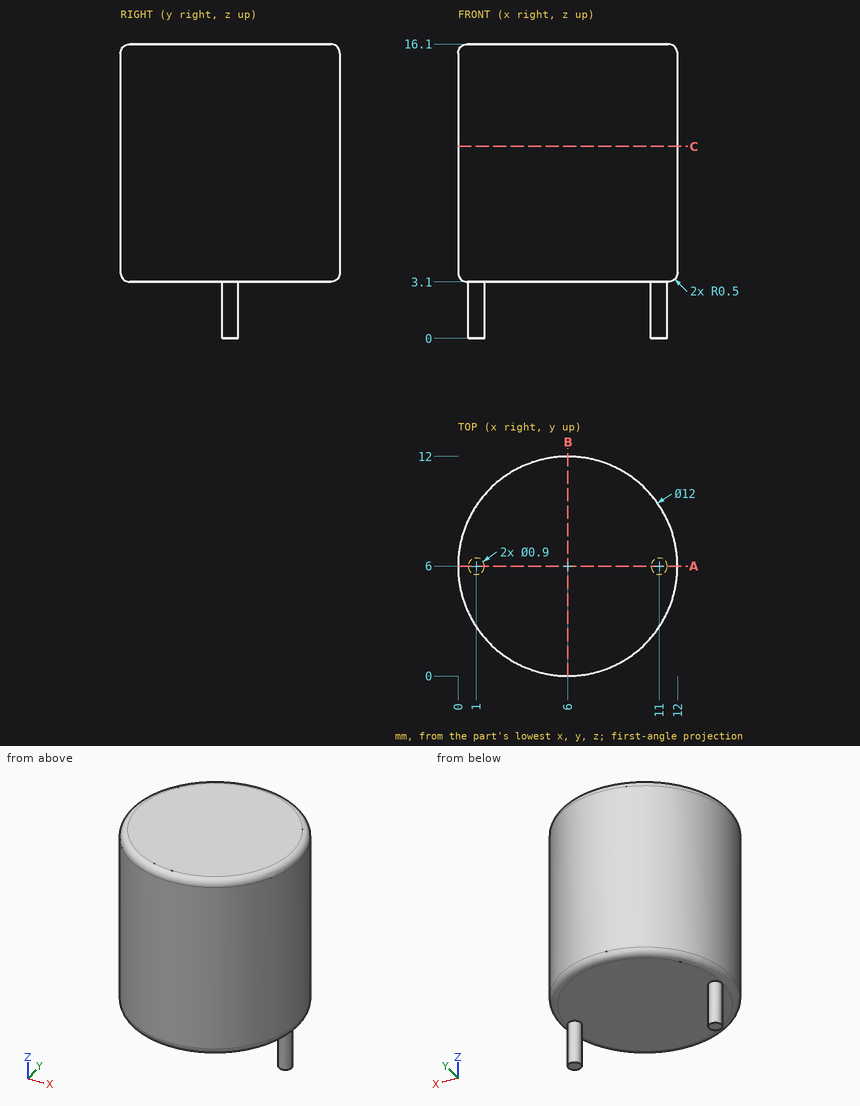
Can you work these out from the drawing? Everything is in mm from the part's minimum corner. Give positions to 0.01 mm unless a question says otherwise; leave off trailing zeros. Loops run counter-clockwise (first coordinate to the right, second up) from the corner with the lowest first, then second, coordinate; pieces in that order, holes last. Notation, with made-up numbers: (58.25, 15) - (82.25, 15) arc R23 ccw to (82.25, 40) - close; hole circle Ø3 at (-22, 54.25). An arc over 180 degrees is marked (long way). Answer as a JSON object with one key per item and string values.
Q1. Imagine slicing it at A-A on y = 6. Write out the boundary of the cut face in (x, z).
Geometry says:
{"outline": "(0, 3.6) arc R0.5 ccw to (0.5, 3.1) - (0.55, 3.1) - (0.55, 0) - (1.45, 0) - (1.45, 3.1) - (10.55, 3.1) - (10.55, 0) - (11.45, 0) - (11.45, 3.1) - (11.5, 3.1) arc R0.5 ccw to (12, 3.6) - (12, 15.6) arc R0.5 ccw to (11.5, 16.1) - (0.5, 16.1) arc R0.5 ccw to (0, 15.6) - close"}
Q2. Will these pins go through, and if not, where does the flat tip stop? P1, Ø1, axis at y = 8, z = 9, coming from the -X side; P2, Ø1.5, axis at x = 3, z = 4, coming from the +Y side; P3, Ø5, axis at y = 2.5, z = 2, coming from the +X side.
Geometry says:
{"P1": "x = 0.19", "P2": "y = 11.56", "P3": "x = 11.8"}
Q3. If I drill on L1, parallel to Z at x = 3, y = 3; L2, parallel to Y at x = 8.5, z = 11; L3, parallel to Y at x = 5.75, z = 5.75, over which ranges is the centre line in solid material (lowest first)?
Geometry says:
{"L1": "3.1 to 16.1", "L2": "0.55 to 11.45", "L3": "0.01 to 11.99"}
Q4. Imagine slicing it at B-B on x = 6. Write out the boundary of the cut face in (y, z), plus the area to 3 significant figures.
Geometry says:
{"outline": "(0, 3.6) arc R0.5 ccw to (0.5, 3.1) - (11.5, 3.1) arc R0.5 ccw to (12, 3.6) - (12, 15.6) arc R0.5 ccw to (11.5, 16.1) - (0.5, 16.1) arc R0.5 ccw to (0, 15.6) - close", "area": "156 mm²"}
Q5. Imagine slicing it at C-C on z = 10.5. Write out the boundary of the cut face in (x, y).
Geometry says:
{"outline": "circle Ø12 at (6, 6)"}
